```python
from build123d import *

# Parameters (mm, degrees)
F1_DEPTH = 9.525


with BuildPart() as f1:
    # F0 (on Front) → F1 (new body, symmetric)
    with BuildSketch(Plane.XZ):
        with BuildLine():
            Line((-19.05, 15.875), (-19.05, 0))
            Line((-19.05, 0), (-9.525, 0))
            ThreePointArc((-9.525, 0), (-6.735192, 6.735192), (0, 9.525))
            ThreePointArc((0, 9.525), (6.735192, 6.735192), (9.525, 0))
            Line((9.525, 0), (19.05, 0))
            Line((19.05, 0), (19.05, 15.875))
            Line((19.05, 15.875), (0, 15.875))
            Line((0, 15.875), (-19.05, 15.875))
        make_face()
    extrude(amount=F1_DEPTH, both=True)


solid = f1.part
```
Verification items for the finished model (mm, model axes). Round coordinates to 2 decimals unless told otherwise and drop trailing zeros. Write each loop counter-clockwise with the first axis right and the second up, starting at its lowest first coordinate (ties: lowest second). Pieces come first, ordered by that corner, then holes.
1. Section check B-B on y = -7.75. Enter the section's corners in (x, z) (3 decimals).
2. Section check C-C on z = 4.5. Enter the section's corners in (x, y) (3 decimals).
3. Scan lines: L1, parallel to X at y = -7, z = 4.25; L2, parallel to X at y = 0.75, z = 1.75; L3, parallel to Z at x = -4, y = -7 (3 decimals). Record each from-to range of solid material in increasing order.
4. Section check A-A on z = 8.25. Enter the section's corners in (x, y) (3 decimals), plus the area to 3 significant figures.
5. Section check D-D on x = -3. Enter the section's corners in (y, z) (3 decimals).
Answer:
1. outline: (-19.05, 0) - (-9.525, 0) arc R9.525 cw to (9.525, 0) - (19.05, 0) - (19.05, 15.875) - (-19.05, 15.875) - close
2. outline: (-19.05, -9.525) - (-8.395, -9.525) - (-8.395, 9.525) - (-19.05, 9.525) - close; (8.395, -9.525) - (19.05, -9.525) - (19.05, 9.525) - (8.395, 9.525) - close
3. L1: x = -19.05 to -8.52, 8.52 to 19.05
3. L2: x = -19.05 to -9.36, 9.36 to 19.05
3. L3: z = 8.644 to 15.875
4. outline: (-19.05, -9.525) - (-4.761, -9.525) - (-4.761, 9.525) - (-19.05, 9.525) - close; (4.761, -9.525) - (19.05, -9.525) - (19.05, 9.525) - (4.761, 9.525) - close
4. area: 544 mm2
5. outline: (-9.525, 9.04) - (9.525, 9.04) - (9.525, 15.875) - (-9.525, 15.875) - close
